from build123d import *

# Parameters (mm, degrees)
AUFSATZ_LINEAR_AUSTRAGEN1_DEPTH = 10
AUFSATZ_LINEAR_AUSTRAGEN1_TAPER = 45
SCHNITT_LINEAR_AUSTRAGEN1_DEPTH = 10
SCHNITT_LINEAR_AUSTRAGEN1_DRAFT = -45
SKIZZE4_W                       = 18.456831932
SKIZZE4_H                       = 18.61324181
SCHNITT_LINEAR_AUSTRAGEN2_DEPTH = 1
LINEAR_AUSTRAGEN_D_NN1_DEPTH    = 2
SKIZZE6_W                       = 1
SKIZZE6_H                       = 2.884303542
SKIZZE6_H_2                     = 4.096110591
AUFSATZ_LINEAR_AUSTRAGEN2_DEPTH = 1.5


with BuildPart() as part:
    # Skizze1 → Aufsatz-Linear austragen1 (new body)
    with BuildSketch(Plane.XY):
        Polygon((0, 18), (-15.588457268, 9), (-15.588457268, -9), (0, -18), (15.588457268, -9), (15.588457268, 9), align=None)
    extrude(amount=AUFSATZ_LINEAR_AUSTRAGEN1_DEPTH, taper=AUFSATZ_LINEAR_AUSTRAGEN1_TAPER)


with BuildPart() as schnitt_linear_austragen1_tool:
    # Skizze3 → Schnitt-Linear austragen1 (with draft: the straight prism first)
    with BuildSketch(Plane(origin=(0, 0, 0), x_dir=(-1, 0, 0), z_dir=(0, 0, -1))):
        Polygon((0, -16.845299462), (14.588457268, -8.422649731), (14.588457268, 8.422649731), (0, 16.845299462), (-14.588457268, 8.422649731), (-14.588457268, -8.422649731), align=None)
    extrude(amount=-SCHNITT_LINEAR_AUSTRAGEN1_DEPTH)
    # Schnitt-Linear austragen1: the draft: its side faces are tilted about the plane it starts from
    schnitt_linear_austragen1_sides = [schnitt_linear_austragen1_tool.faces().sort_by_distance(p)[0] for p in [
        (-7.294228634, -12.633974596, 5),
        (-14.588457268, 0, 5),
        (-7.294228634, 12.633974596, 5),
        (7.294228634, 12.633974596, 5),
        (14.588457268, 0, 5),
        (7.294228634, -12.633974596, 5),
    ]]
    draft(schnitt_linear_austragen1_sides, Plane(origin=(0, 0, 0), x_dir=(-1, 0, 0), z_dir=(0, 0, -1)), SCHNITT_LINEAR_AUSTRAGEN1_DRAFT)


with BuildPart() as part_1:
    add(part.part)

    # Schnitt-Linear austragen1: cut by schnitt_linear_austragen1_tool
    add(schnitt_linear_austragen1_tool.part, mode=Mode.SUBTRACT)

    # Skizze4 → Schnitt-Linear austragen2 (cut)
    with BuildSketch(Plane.XY.offset(10)):
        with Locations((-0.579719129, -0.066676412)):
            Rectangle(SKIZZE4_W, SKIZZE4_H)
    extrude(amount=-SCHNITT_LINEAR_AUSTRAGEN2_DEPTH, mode=Mode.SUBTRACT)

    # Skizze5 → Linear-Austragen-Dünn1 (add)
    with BuildSketch(Plane(origin=(0, 0, 0), x_dir=(-1, 0, 0), z_dir=(0, 0, -1))):
        Polygon((0, 18), (-15.588457268, 9), (-15.588457268, -9), (0, -18), (15.588457268, -9), (15.588457268, 9), align=None)
        Polygon((0, 16.845299462), (-14.588457268, 8.422649731), (-14.588457268, -8.422649731), (0, -16.845299462), (14.588457268, -8.422649731), (14.588457268, 8.422649731), align=None, mode=Mode.SUBTRACT)
    extrude(amount=LINEAR_AUSTRAGEN_D_NN1_DEPTH)

    # Skizze6 → Aufsatz-Linear austragen2 (add)
    with BuildSketch(Plane.XY.offset(9)):
        Polygon((-4.749990863, 4.865286651), (-4.249990863, 3.999261247), (-1.59539386, 5.531893541), (-2.09539386, 6.397918945), align=None)
        Polygon((1.921657415, 6.498225729), (1.421657415, 5.632200325), (3.989719656, 4.149528899), (4.489719656, 5.015554303), align=None)
        with Locations((6.088457268, -0.039837206)):
            Rectangle(SKIZZE6_W, SKIZZE6_H)
        Polygon((4.739719656, -4.871216735), (4.239719656, -4.005191332), (0.921657415, -5.92087546), (1.421657415, -6.786900863), align=None)
        Polygon((-1.421657415, -6.786900863), (-0.921657415, -5.92087546), (-4.48199319, -3.865314642), (-4.98199319, -4.731340045), align=None)
        with Locations((-6.088457268, -0.132397801)):
            Rectangle(SKIZZE6_W, SKIZZE6_H_2)
    extrude(amount=AUFSATZ_LINEAR_AUSTRAGEN2_DEPTH)


solid = part_1.part
Could you check a few things on this model? Use its own coordinates, in mm. A direction names the side the tool comes from. Round coordinates to 2 decimals unless told otherwise and drop trailing zeros. Loops run counter-clockwise (first coordinate to the right, second up) from the corner with the lowest first, then second, coordinate; pieces in that order, holes last. Notation, with made-up numbers: (16.25, -38.5) - (66.25, -38.5) arc R33 cw to (66.25, -6.5) - close; hole circle Ø6 at (-35.75, 54). An arc over 180 degrees is marked (long way). Write item = value, one per line.
1) I'm going to push flat-ended pins straight in: P1, Ø0.6, axis at x = 0.5, y = 6.5, coming from the +Z side; P2, Ø1, axis at x = 3, y = -14, coming from the +Z side; P3, Ø1.6, axis at y = 0.5, z = 9.5, coming from the -X side. Where does each tip first touch, or does it pass through?
Computed:
P1 = 9
P2 = 2.46
P3 = -6.89
2) If we mould it in two halves opening along Y, with no side actions, what happens to faces 1 (the flat face through (14.588, 0, -1)), 2 (the flat face through (3, -5, 10.5)), 3 (the flat face through (2.69, 4.9, 9.74)), 4 (the flat face through (-6.18, 10.46, 3.44))? For each: pulls with the +Y half, pulls with the -Y half, needs draft (parallel to the pull), parting line crosses it, or undercut.
Computed:
face_1 = undercut
face_2 = needs draft
face_3 = undercut
face_4 = pulls with the +Y half
3) Imagine slicing it at B-B (y = 0.5). Please give me the cut outline in (x, z).
Computed:
outline = (-15.59, -2) - (-14.59, -2) - (-14.59, 0) - (-5.59, 9) - (-5.59, 10.5) - (-6.59, 10.5) - (-6.59, 9) - (-15.59, 0) - close; (5.59, 9) - (14.59, 0) - (14.59, -2) - (15.59, -2) - (15.59, 0) - (6.59, 9) - (6.59, 10.5) - (5.59, 10.5) - close
4) Imagine slicing it at D-D (z = 7.25). Please give me the cut outline in (x, y), and give its area (3 significant figures).
Computed:
outline = (-8.34, -4.81) - (0, -9.63) - (8.34, -4.81) - (8.34, 4.81) - (0, 9.63) - (-8.34, 4.81) - close; hole (-7.34, -4.24) - (0, -8.47) - (7.34, -4.24) - (7.34, 4.24) - (0, 8.47) - (-7.34, 4.24) - close
area = 54.3 mm2
5) Imagine slicing it at C-C (x = 9.5). Please give me the cut outline in (y, z), and give its area (3 significant figures).
Computed:
outline = (-12.52, -2) - (-11.36, -2) - (-11.36, 0) - (-5.48, 5.09) - (5.48, 5.09) - (11.36, 0) - (11.36, -2) - (12.52, -2) - (12.52, 0) - (5.48, 6.09) - (-5.48, 6.09) - (-12.52, 0) - close
area = 28.5 mm2
6) I need wall thicknesses on line 1 along Y through (x, z) = (10, -0.5); line 2 along X through (y, z) = (7, 4); line 3 along Y through (x, z) = (-4, 6). Which ranges of each line are inside material? Lowest first, please. Write a range as from..to.
Computed:
line_1 = -12.23..-11.07, 11.07..12.23
line_2 = -11.05..-9.05, 9.05..11.05
line_3 = -8.76..-7.61, 7.61..8.76
7) Imagine slicing it at A-A (z = -0.75). Please give me the cut outline in (x, y), and give its area (3 significant figures).
Computed:
outline = (-15.59, -9) - (0, -18) - (15.59, -9) - (15.59, 9) - (0, 18) - (-15.59, 9) - close; hole (-14.59, -8.42) - (0, -16.85) - (14.59, -8.42) - (14.59, 8.42) - (0, 16.85) - (-14.59, 8.42) - close
area = 105 mm2
8) On a 3-axis mill with a long thin cutter (end or side, diameter ignored), from which of +Z, -Z, +X, -X, +Y, -Y can I reach the whole of each face in a straight line? I mean faces 5 (the flat face through (5.588, 0, 10)), 6 (the flat face through (6.588, 0, 10)), 7 (the flat face through (-6.588, 0, 10)). Say none if no direction works.
Computed:
face_5 = +Z, -Z, +Y, -Y
face_6 = +Z, +X, +Y, -Y
face_7 = +Z, -X, +Y, -Y
